from build123d import *

# Parameters (mm, degrees)
F0_R         = 52.451
F0_R_2       = 39.751
F1_DEPTH     = 25.4
F3_DEPTH     = 50.8
F4_T4_ANGLE  = 145.1483416982
F4_T9_ANGLE  = 145.1483416982
F4_T16_ANGLE = 145.1483416982
F4_T23_ANGLE = 145.1483416982
F4_T28_ANGLE = 42.5640131775
F4_T33_ANGLE = 42.5640131775
F4_T38_ANGLE = 102.5699239424
F4_T44_ANGLE = 102.5699239424
F4_T49_ANGLE = 102.5699239424
F4_T54_ANGLE = 145.1483416982
F4_T59_ANGLE = 145.1483416982
F4_T66_ANGLE = 145.1483416982
F4_T73_ANGLE = 145.1483416982


# Not quite as in the source:
# - a fillet or chamfer that OpenCascade refuses, or shapes differently, is made with other operations: its cross-section is extruded or revolved along the edge and cut away or added


with BuildPart() as f1:
    # F0 (on Top) → F1 (new body)
    with BuildSketch(Plane.XY):
        Circle(F0_R)
        Circle(F0_R_2, mode=Mode.SUBTRACT)
    extrude(amount=F1_DEPTH)

    # F2 (on face) → F3 (join)
    with BuildSketch(Plane.XY.offset(25.4)):
        Polygon((0, 39.751), (3.9769716214, 39.5515574627), (8.3683463891, 51.7791288041), (0, 52.451), (-8.3683463891, 51.7791288041), (-3.9769716214, 39.5515574627), align=None)
        Polygon((-49.0262141247, -18.6423638414), (-45.4238984539, -26.2255), (-40.6578677356, -33.1367649627), (-32.2641677112, -23.2199371856), (-34.4253758258, -19.8755), (-36.2411393326, -16.331620277), align=None)
        Polygon((40.6578677356, -33.1367649627), (45.4238984539, -26.2255), (49.0262141247, -18.6423638414), (36.2411393326, -16.331620277), (34.4253758258, -19.8755), (32.2641677112, -23.2199371856), align=None)
    extrude(amount=F3_DEPTH)

    # F4: fillet of radius 5.08 on 4 edges, made by hand


with BuildPart() as f4_tool2:
    # F4_s3 → F4_t4 (revolve)
    with BuildSketch(Plane(origin=(0, 0, 0), x_dir=(0, 0, 1), z_dir=(0.9760150026, -0.2177032723, 0))):
        with BuildLine():
            ThreePointArc((25.4, -44.831), (23.9121024484, -41.2388975516), (20.32, -39.751))
            Line((20.32, -39.751), (25.4, -39.751))
            Line((25.4, -39.751), (25.4, -44.831))
        make_face()
    revolve(axis=Axis((0, 0, 25.4), (0, 0, 1)), revolution_arc=F4_T4_ANGLE)

    split(bisect_by=Plane(origin=(-9.0590317285, 3.2534345735, 0), x_dir=(0, 0, 1), z_dir=(0.9411459494, -0.3380004466, 0)), keep=Keep.TOP)


with BuildPart() as f1_1:
    add(f1.part)

    # F4_t1: cut F4_tool2
    add(f4_tool2.part, mode=Mode.SUBTRACT)


with BuildPart() as f4_tool7:
    # F4_s8 → F4_t9 (revolve)
    with BuildSketch(Plane(origin=(0, 0, 0), x_dir=(0, 0, 1), z_dir=(0.9760150026, -0.2177032723, 0))):
        with BuildLine():
            ThreePointArc((25.4, -44.831), (23.9121024484, -41.2388975516), (20.32, -39.751))
            Line((20.32, -39.751), (25.4, -39.751))
            Line((25.4, -39.751), (25.4, -44.831))
        make_face()
    revolve(axis=Axis((0, 0, 25.4), (0, 0, 1)), revolution_arc=F4_T9_ANGLE)

    split(bisect_by=Plane(origin=(9.0590317285, 3.2534345735, 0), x_dir=(0, 0, 1), z_dir=(-0.9411459494, -0.3380004466, 0)), keep=Keep.TOP)

    split(bisect_by=Plane(origin=(-33.3447717685, -21.5477185928, 0), x_dir=(0, 0, 1), z_dir=(0.8398952423, 0.542748544, 0)), keep=Keep.TOP)

    split(bisect_by=Plane(origin=(-35.3332575792, -18.1035601385, 0), x_dir=(0, 0, 1), z_dir=(0.8899816481, 0.4559963443, 0)), keep=Keep.TOP)


with BuildPart() as f1_2:
    add(f1_1.part)

    # F4_t6: cut F4_tool7
    add(f4_tool7.part, mode=Mode.SUBTRACT)


with BuildPart() as f4_tool14:
    # F4_s15 → F4_t16 (revolve)
    with BuildSketch(Plane(origin=(0, 0, 0), x_dir=(0, 0, 1), z_dir=(0.9760150026, -0.2177032723, 0))):
        with BuildLine():
            ThreePointArc((25.4, -44.831), (23.9121024484, -41.2388975516), (20.32, -39.751))
            Line((20.32, -39.751), (25.4, -39.751))
            Line((25.4, -39.751), (25.4, -44.831))
        make_face()
    revolve(axis=Axis((0, 0, 25.4), (0, 0, 1)), revolution_arc=F4_T16_ANGLE)

    split(bisect_by=Plane(origin=(1.7119588741, -9.4720688973, 0), x_dir=(0, 0, 1), z_dir=(-0.1778560014, 0.9840565242, 0)), keep=Keep.TOP)

    split(bisect_by=Plane(origin=(1.9884858107, 39.6512787313, 0), x_dir=(0, 0, 1), z_dir=(-0.0500864058, -0.9987448883, 0)), keep=Keep.TOP)

    split(bisect_by=Plane(origin=(-1.9884858107, 39.6512787313, 0), x_dir=(0, 0, 1), z_dir=(0.0500864058, -0.9987448883, 0)), keep=Keep.TOP)


with BuildPart() as f1_3:
    add(f1_2.part)

    # F4_t13: cut F4_tool14
    add(f4_tool14.part, mode=Mode.SUBTRACT)


with BuildPart() as f4_tool21:
    # F4_s22 → F4_t23 (revolve)
    with BuildSketch(Plane(origin=(0, 0, 0), x_dir=(0, 0, 1), z_dir=(0.9760150026, -0.2177032723, 0))):
        with BuildLine():
            ThreePointArc((25.4, -44.831), (23.9121024484, -41.2388975516), (20.32, -39.751))
            Line((20.32, -39.751), (25.4, -39.751))
            Line((25.4, -39.751), (25.4, -44.831))
        make_face()
    revolve(axis=Axis((0, 0, 25.4), (0, 0, 1)), revolution_arc=F4_T23_ANGLE)

    split(bisect_by=Plane(origin=(-7.3470728544, 6.2186343238, 0), x_dir=(0, 0, 1), z_dir=(0.763289948, -0.6460560775, 0)), keep=Keep.TOP)


with BuildPart() as f1_4:
    add(f1_3.part)

    # F4_t20: cut F4_tool21
    add(f4_tool21.part, mode=Mode.SUBTRACT)


with BuildPart() as f4_tool26:
    # F4_s27 → F4_t28 (revolve)
    with BuildSketch(Plane(origin=(0, 0, 0), x_dir=(0, 0, 1), z_dir=(-0.6764135021, -0.7365220799, 0))):
        with BuildLine():
            ThreePointArc((25.4, -44.831), (23.9121024484, -41.2388975516), (20.32, -39.751))
            Line((20.32, -39.751), (25.4, -39.751))
            Line((25.4, -39.751), (25.4, -44.831))
        make_face()
    revolve(axis=Axis((0, 0, 25.4), (0, 0, 1)), revolution_arc=F4_T28_ANGLE)

    split(bisect_by=Plane(origin=(7.3470728544, 6.2186343238, 0), x_dir=(0, 0, 1), z_dir=(-0.763289948, -0.6460560775, 0)), keep=Keep.TOP)


with BuildPart() as f1_5:
    add(f1_4.part)

    # F4_t25: cut F4_tool26
    add(f4_tool26.part, mode=Mode.SUBTRACT)


with BuildPart() as f4_tool31:
    # F4_s32 → F4_t33 (revolve)
    with BuildSketch(Plane(origin=(0, 0, 0), x_dir=(0, 0, 1), z_dir=(-0.6764135021, -0.7365220799, 0))):
        with BuildLine():
            ThreePointArc((25.4, -44.831), (23.9121024484, -41.2388975516), (20.32, -39.751))
            Line((20.32, -39.751), (25.4, -39.751))
            Line((25.4, -39.751), (25.4, -44.831))
        make_face()
    revolve(axis=Axis((0, 0, 25.4), (0, 0, 1)), revolution_arc=F4_T33_ANGLE)

    split(bisect_by=Plane(origin=(-1.7119588741, -9.4720688973, 0), x_dir=(0, 0, 1), z_dir=(0.1778560014, 0.9840565242, 0)), keep=Keep.TOP)


with BuildPart() as f1_6:
    add(f1_5.part)

    # F4_t30: cut F4_tool31
    add(f4_tool31.part, mode=Mode.SUBTRACT)


with BuildPart() as f4_tool36:
    # F4_s37 → F4_t38 (revolve)
    with BuildSketch(Plane.XZ):
        with BuildLine():
            ThreePointArc((44.831, 25.4), (41.2388975516, 23.9121024484), (39.751, 20.32))
            Line((39.751, 20.32), (39.751, 25.4))
            Line((39.751, 25.4), (44.831, 25.4))
        make_face()
    revolve(axis=Axis((0, 0, 25.4), (0, 0, 1)), revolution_arc=F4_T38_ANGLE)

    split(bisect_by=Plane(origin=(1.9884858107, 39.6512787313, 0), x_dir=(0, 0, 1), z_dir=(-0.0500864058, -0.9987448883, 0)), keep=Keep.TOP)

    split(bisect_by=Plane(origin=(-1.9884858107, 39.6512787313, 0), x_dir=(0, 0, 1), z_dir=(0.0500864058, -0.9987448883, 0)), keep=Keep.TOP)


with BuildPart() as f1_7:
    add(f1_6.part)

    # F4_t35: cut F4_tool36
    add(f4_tool36.part, mode=Mode.SUBTRACT)


with BuildPart() as f4_tool42:
    # F4_s43 → F4_t44 (revolve)
    with BuildSketch(Plane.XZ):
        with BuildLine():
            ThreePointArc((44.831, 25.4), (41.2388975516, 23.9121024484), (39.751, 20.32))
            Line((39.751, 20.32), (39.751, 25.4))
            Line((39.751, 25.4), (44.831, 25.4))
        make_face()
    revolve(axis=Axis((0, 0, 25.4), (0, 0, 1)), revolution_arc=F4_T44_ANGLE)

    split(bisect_by=Plane(origin=(-9.0590317285, 3.2534345735, 0), x_dir=(0, 0, 1), z_dir=(0.9411459494, -0.3380004466, 0)), keep=Keep.TOP)


with BuildPart() as f1_8:
    add(f1_7.part)

    # F4_t41: cut F4_tool42
    add(f4_tool42.part, mode=Mode.SUBTRACT)


with BuildPart() as f4_tool47:
    # F4_s48 → F4_t49 (revolve)
    with BuildSketch(Plane.XZ):
        with BuildLine():
            ThreePointArc((44.831, 25.4), (41.2388975516, 23.9121024484), (39.751, 20.32))
            Line((39.751, 20.32), (39.751, 25.4))
            Line((39.751, 25.4), (44.831, 25.4))
        make_face()
    revolve(axis=Axis((0, 0, 25.4), (0, 0, 1)), revolution_arc=F4_T49_ANGLE)

    split(bisect_by=Plane(origin=(9.0590317285, 3.2534345735, 0), x_dir=(0, 0, 1), z_dir=(-0.9411459494, -0.3380004466, 0)), keep=Keep.TOP)


with BuildPart() as f1_9:
    add(f1_8.part)

    # F4_t46: cut F4_tool47
    add(f4_tool47.part, mode=Mode.SUBTRACT)


with BuildPart() as f4_tool52:
    # F4_s53 → F4_t54 (revolve)
    with BuildSketch(Plane(origin=(0, 0, 0), x_dir=(0, 0, 1), z_dir=(-0.299470937, 0.9541054229, 0))):
        with BuildLine():
            ThreePointArc((25.4, -44.831), (23.9121024484, -41.2388975516), (20.32, -39.751))
            Line((20.32, -39.751), (25.4, -39.751))
            Line((25.4, -39.751), (25.4, -44.831))
        make_face()
    revolve(axis=Axis((0, 0, 25.4), (0, 0, 1)), revolution_arc=F4_T54_ANGLE)

    split(bisect_by=Plane(origin=(1.7119588741, -9.4720688973, 0), x_dir=(0, 0, 1), z_dir=(-0.1778560014, 0.9840565242, 0)), keep=Keep.TOP)


with BuildPart() as f1_10:
    add(f1_9.part)

    # F4_t51: cut F4_tool52
    add(f4_tool52.part, mode=Mode.SUBTRACT)


with BuildPart() as f4_tool57:
    # F4_s58 → F4_t59 (revolve)
    with BuildSketch(Plane(origin=(0, 0, 0), x_dir=(0, 0, 1), z_dir=(-0.299470937, 0.9541054229, 0))):
        with BuildLine():
            ThreePointArc((25.4, -44.831), (23.9121024484, -41.2388975516), (20.32, -39.751))
            Line((20.32, -39.751), (25.4, -39.751))
            Line((25.4, -39.751), (25.4, -44.831))
        make_face()
    revolve(axis=Axis((0, 0, 25.4), (0, 0, 1)), revolution_arc=F4_T59_ANGLE)

    split(bisect_by=Plane(origin=(-7.3470728544, 6.2186343238, 0), x_dir=(0, 0, 1), z_dir=(0.763289948, -0.6460560775, 0)), keep=Keep.TOP)

    split(bisect_by=Plane(origin=(35.3332575792, -18.1035601385, 0), x_dir=(0, 0, 1), z_dir=(-0.8899816481, 0.4559963443, 0)), keep=Keep.TOP)

    split(bisect_by=Plane(origin=(33.3447717685, -21.5477185928, 0), x_dir=(0, 0, 1), z_dir=(-0.8398952423, 0.542748544, 0)), keep=Keep.TOP)


with BuildPart() as f1_11:
    add(f1_10.part)

    # F4_t56: cut F4_tool57
    add(f4_tool57.part, mode=Mode.SUBTRACT)


with BuildPart() as f4_tool64:
    # F4_s65 → F4_t66 (revolve)
    with BuildSketch(Plane(origin=(0, 0, 0), x_dir=(0, 0, 1), z_dir=(-0.299470937, 0.9541054229, 0))):
        with BuildLine():
            ThreePointArc((25.4, -44.831), (23.9121024484, -41.2388975516), (20.32, -39.751))
            Line((20.32, -39.751), (25.4, -39.751))
            Line((25.4, -39.751), (25.4, -44.831))
        make_face()
    revolve(axis=Axis((0, 0, 25.4), (0, 0, 1)), revolution_arc=F4_T66_ANGLE)

    split(bisect_by=Plane(origin=(7.3470728544, 6.2186343238, 0), x_dir=(0, 0, 1), z_dir=(-0.763289948, -0.6460560775, 0)), keep=Keep.TOP)

    split(bisect_by=Plane(origin=(-33.3447717685, -21.5477185928, 0), x_dir=(0, 0, 1), z_dir=(0.8398952423, 0.542748544, 0)), keep=Keep.TOP)

    split(bisect_by=Plane(origin=(-35.3332575792, -18.1035601385, 0), x_dir=(0, 0, 1), z_dir=(0.8899816481, 0.4559963443, 0)), keep=Keep.TOP)


with BuildPart() as f1_12:
    add(f1_11.part)

    # F4_t63: cut F4_tool64
    add(f4_tool64.part, mode=Mode.SUBTRACT)


with BuildPart() as f4_tool71:
    # F4_s72 → F4_t73 (revolve)
    with BuildSketch(Plane(origin=(0, 0, 0), x_dir=(0, 0, 1), z_dir=(-0.299470937, 0.9541054229, 0))):
        with BuildLine():
            ThreePointArc((25.4, -44.831), (23.9121024484, -41.2388975516), (20.32, -39.751))
            Line((20.32, -39.751), (25.4, -39.751))
            Line((25.4, -39.751), (25.4, -44.831))
        make_face()
    revolve(axis=Axis((0, 0, 25.4), (0, 0, 1)), revolution_arc=F4_T73_ANGLE)

    split(bisect_by=Plane(origin=(-1.7119588741, -9.4720688973, 0), x_dir=(0, 0, 1), z_dir=(0.1778560014, 0.9840565242, 0)), keep=Keep.TOP)


with BuildPart() as f1_13:
    add(f1_12.part)

    # F4_t70: cut F4_tool71
    add(f4_tool71.part, mode=Mode.SUBTRACT)


solid = f1_13.part
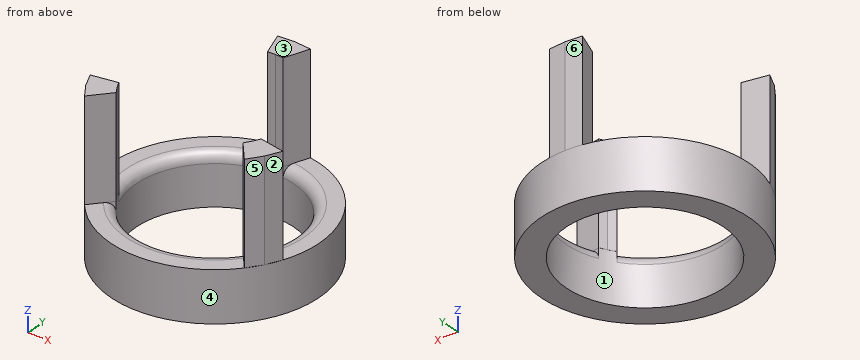
Here's how the part is built. I have some questions about the finished solid (model axes, mm). Face numbers are marked on the shaded views. A direction names the side the tool comes from. Give positions to 0.01 mm unless a question says otherwise; leave off trailing zeros. Order: outer loops, then holes, each group sorted by start corner. A loop starts at its lowest first (then second) coordinate and runs counter-clockwise, first axis right, second up. Notation, with made-up numbers: M 88.5,20 L 118.5,20 A10 ccw 118.5,38 Z; hole C 60,-30 d10. An arc over 180 degrees is marked long. Answer as a JSON object with one key per item and string values. Group by question number.
1) Suppose I cut it at A-A, the plane z = 43.5. Write out the boundary of the cut face in (x, y).
2) I'm going to push flat-ended pins straight in: pin 1 Ø7.5 at (x, y) = (1.5, -41.5) entering from +Z; pin 2 Ø1.5 at (x, z) = (-32.5, 33.5) entering from -Y; pin 3 Ø5 at (x, z) = (20, 24.5) entering from +Y; pin 4 Ø0.6 at (x, y) = (34, -21) entering from -Z. Where does each tip first touch, or does it pass through?
3) We'd pull the mould along X, two halves only. Please class the marked faces 1, 2 and 3: pulls with the +X half, pulls with the -X half, needs draft (parallel to the pull), parting line crosses it, or undercut.
4) On a 3-axis mill with a long thin cutter (end or side, diameter ignored), from which of +Z, -Z, +X, -X, +Y, -Y can I reach the whole of each face in a straight line? I mean the marked faces 4, 5 and 6. Say none if no direction works.
5) Suppose I cut it at B-B, the plane y = 0. Write out the boundary of the cut face in (x, z), plus the area to 3 significant figures.
6) Please list where this line runs through material, in increasing order: L1, parallel to Y at x = 0, z = 14. Write a range as [from, to].
7) Suppose I cut it at C-C, the plane z = 15.5. Write out the boundary of the cut face in (x, y), plus the area to 3 significant figures.
Results found:
{
 "1": {"outline": "M -49.03,-18.64 L -45.42,-26.23 L -40.66,-33.14 L -32.26,-23.22 L -34.43,-19.88 L -36.24,-16.33 Z; M -8.37,51.78 L -3.98,39.55 L 0,39.75 L 3.98,39.55 L 8.37,51.78 L 0,52.45 Z; M 32.26,-23.22 L 40.66,-33.14 L 45.42,-26.23 L 49.03,-18.64 L 36.24,-16.33 L 34.43,-19.88 Z"},
 "2": {"pin 1": "z = 25.4", "pin 2": "y = -24.38", "pin 3": "y = 49.45", "pin 4": "z = 0"},
 "3": {"face 1": "undercut", "face 2": "pulls with the +X half", "face 3": "needs draft"},
 "4": {"face 4": "+Z, -Z", "face 5": "+Z, +X, -Y", "face 6": "+Z, -X, +Y"},
 "5": {"outline": "M -52.45,0 L -39.75,0 L -39.75,20.32 A5.08 ccw -44.83,25.4 L -52.45,25.4 Z; M 39.75,0 L 52.45,0 L 52.45,25.4 L 44.83,25.4 A5.08 ccw 39.75,20.32 Z", "area": "634 mm²"},
 "6": {"L1": "[-52.45, -39.75], [39.75, 52.45]"},
 "7": {"outline": "C 0,0 d104.9; hole C 0,0 d79.5", "area": "3,680 mm²"}
}
